from build123d import *

# Parameters (mm, degrees)
SKETCH1_R               = 7.5
BOSS_EXTRUDE1_DEPTH     = 10
BOSS_EXTRUDE2_OUTLINE_R = 7.5
BOSS_EXTRUDE2_DEPTH     = 9


# Read off the part's stored shape, not the designer's step: Boss-Extrude2
with BuildPart() as part:
    # Sketch1 → Boss-Extrude1 (new body)
    with BuildSketch(Plane(origin=(0, 0, 0), x_dir=(1, 0, 0), z_dir=(0, 1, 0))):
        with BuildLine():
            Line((-6, 23), (-6, 23.237900077))
            ThreePointArc((-6, 23.237900077), (0, -24), (6, 23.237900077))
            Line((6, 23.237900077), (6, 23))
            Line((6, 23), (6, 11))
            Line((6, 11), (-6, 11))
            Line((-6, 11), (-6, 23))
        make_face()
        with Locations(Location((0, 0, 0), (0, 0, 270))):
            Circle(SKETCH1_R, mode=Mode.SUBTRACT)
    extrude(amount=BOSS_EXTRUDE1_DEPTH)

    # Boss-Extrude2 outline → Boss-Extrude2 (add)
    with BuildSketch(Plane(origin=(0, 0, 0), x_dir=(1, 0, 0), z_dir=(0, 1, 0))):
        Circle(BOSS_EXTRUDE2_OUTLINE_R)
    extrude(amount=BOSS_EXTRUDE2_DEPTH)


solid = part.part
Check sheet for the modelled part. Datum: model origin and axes. Units: mm. A direction names the side the tool comes from. Round coordinates to 2 decimals unless told otherwise and drop trailing zeros. Loops run counter-clockwise (first coordinate to the right, second up) from the corner with the lowest first, then second, coordinate; pieces in that order, holes last. Notation, with made-up numbers: (64, 64.25) -> (108, 64.25) arc R29 cw to (108, 91.25) -> close; hole circle Ø2 at (68, 30.25). An arc over 180 degrees is marked (long way). Put each result on its own line as item: value. Start each with the question number.
1. Gauge pin test, flat ends, axial feed: pin 1 (3 mm diameter, centred on x = 0.5, y = 6.5, fed in from -Z); pin 2 (2 mm diameter, centred on y = 5, z = 1, fed in from +X); pin 3 (2 mm diameter, centred on y = 5.5, z = -3, fed in from +X); pin 4 (5 mm diameter, centred on y = 4.5, z = -16, fed in from -X). Record the tip position at first contact, or that the pin passes through.
2. Section check A-A (z = 0). Enter the section's corners in (x, y).
3. Section check C-C (x = 0). Enter the section's corners in (y, z), plus the area to 3 significant figures.
4. Section check D-D (y = 1). Enter the section's corners in (x, z).
5. Access from +Z, -Z, +X, -X, +Y, -Y to the whole of each face (thin tool, end or side, straight path). Record for faces 5 (the face through (-6, 5, -17)), 6 (the face through (-6, 10, 5)).
6. Scan lines: probe 1 along X at (y, z) = (9.45, 0); probe 2 along X at (y, z) = (3.5, 19); probe 3 along Z at (x, y) = (4, 9.25). Record each from-to range of solid material in increasing order.
7. Draft check along Z on faces 1 (the face through (-0.97, 4.93, 23.98)), 2 (the face through (6, 5, -17)), 3 (the face through (-2.87, 9.49, 6.93)), 4 (the face through (0, 9, 0)). Enter one of: +Z half, -Z half, draft (parallel to the pull), parting line (faces both ways), or undercut.
8. Section check B-B (z = -20). Enter the section's corners in (x, y), plus the area to 3 significant figures.
Findings:
1. pin 1: stops at z = -11
1. pin 2: stops at x = 24
1. pin 3: stops at x = 23.92
1. pin 4: stops at x = -19.84
2. outline: (-24, 0) -> (24, 0) -> (24, 10) -> (7.5, 10) -> (7.5, 9) -> (-7.5, 9) -> (-7.5, 10) -> (-24, 10) -> close
3. outline: (0, -11) -> (10, -11) -> (10, -7.5) -> (9, -7.5) -> (9, 7.5) -> (10, 7.5) -> (10, 24) -> (0, 24) -> close
3. area: 335 mm^2
4. outline: (-6, -23.24) -> (-6, -11) -> (6, -11) -> (6, -23.24) arc R24 ccw (long way) to start
5. face 5: -Z, +Y, -Y
5. face 6: +Z, -Z, +X, -X, +Y
6. probe 1: x = -24 to -7.5, 7.5 to 24
6. probe 2: x = -14.66 to 14.66
6. probe 3: z = -11 to -6.34, 6.34 to 23.66
7. face 1: parting line
7. face 2: draft
7. face 3: undercut
7. face 4: undercut
8. outline: (-13.27, 0) -> (-6, 0) -> (-6, 10) -> (-13.27, 10) -> close; (6, 0) -> (13.27, 0) -> (13.27, 10) -> (6, 10) -> close
8. area: 145 mm^2
